```python
from build123d import *

# Parameters (mm, degrees)
SKETCH_1_W          = 55
SKETCH_1_H          = 40
SKETCH_1_R          = 1.5
EXTRUDE_1_DEPTH     = 3
SKETCH_2_W          = 40
SKETCH_2_H          = 3
EXTRUDE_2_DEPTH     = 4
CUT_EXTRUDE_1_REACH = 39.433
SKETCH_3_R          = 1.5
SKETCH_4_R          = 10.5
EXTRUDE_3_DEPTH     = 5
CUT_EXTRUDE_4_REACH = 40.646
CUT_EXTRUDE_START   = -1
SKETCH_5_W          = 41.614213562
SKETCH_5_H          = 21.814213562
SKETCH_6_R          = 1.5
EXTRUDE_5_DEPTH     = 27
SKETCH_7_W          = 6
SKETCH_7_H          = 25
SKETCH_7_R          = 1.5
EXTRUDE_6_DEPTH     = 8
CUT_EXTRUDE_5_REACH = 70.124
SKETCH_8_W          = 8
SKETCH_8_H          = 7.8
FILLET_1_R          = 3
FILLET_2_R          = 3
CUT_EXTRUDE_START_2 = -5
SKETCH_9_R          = 10.5
CUT_EXTRUDE_6_DEPTH = 5
SKETCH_10_W         = 41.614213562
SKETCH_10_H         = 3
EXTRUDE_7_DEPTH     = 18
FILLET_3_R          = 3
CUT_EXTRUDE_7_REACH = 57.154


with BuildPart() as part:
    # 草图1 → 凸台-拉伸1 (new body)
    with BuildSketch(Plane(origin=(0, 0, 0), x_dir=(1, 0, 0), z_dir=(0, 1, 0))):
        Rectangle(SKETCH_1_W, SKETCH_1_H)
        with Locations(Location((22.3, 5, 0), (0, 0, 270))):
            Circle(SKETCH_1_R, mode=Mode.SUBTRACT)
        with Locations(Location((22.3, -5, 0), (0, 0, 90))):
            Circle(SKETCH_1_R, mode=Mode.SUBTRACT)
    extrude(amount=EXTRUDE_1_DEPTH)

    # 草图2 → 凸台-拉伸2 (add)
    with BuildSketch(Plane.ZY.offset(27.5)):
        with Locations((0, 1.5)):
            Rectangle(SKETCH_2_W, SKETCH_2_H)
    extrude(amount=EXTRUDE_2_DEPTH)

    # 草图3 → 切除-拉伸1 (cut, up to next)
    with BuildSketch(Plane.XZ, mode=Mode.PRIVATE) as cut_extrude_1_sk1:
        with Locations(Location((-27.3, 5, 0), (0, 0, 270))):
            Circle(SKETCH_3_R)
    cut_extrude_1_tool1 = extrude(cut_extrude_1_sk1.sketch, amount=-CUT_EXTRUDE_1_REACH, mode=Mode.PRIVATE) & part.part
    # 草图3 → 切除-拉伸1 (cut, up to next)
    with BuildSketch(Plane.XZ, mode=Mode.PRIVATE) as cut_extrude_1_sk2:
        with Locations(Location((-27.3, -5, 0), (0, 0, 270))):
            Circle(SKETCH_3_R)
    cut_extrude_1_tool2 = extrude(cut_extrude_1_sk2.sketch, amount=-CUT_EXTRUDE_1_REACH, mode=Mode.PRIVATE) & part.part
    add(cut_extrude_1_tool1.solids().sort_by_distance((-27.3, 0, 5))[0], mode=Mode.SUBTRACT)
    add(cut_extrude_1_tool2.solids().sort_by_distance((-27.3, 0, -5))[0], mode=Mode.SUBTRACT)

    # 草图4 → 凸台-拉伸3 (add)
    with BuildSketch(Plane.XZ):
        with Locations(Location((-12.5, 0, 0), (0, 0, 90))):
            Circle(SKETCH_4_R)
    extrude(amount=EXTRUDE_3_DEPTH)

    # 草图5 → 切除-拉伸4 (cut, up to next)
    with BuildSketch(Plane.XZ.offset(CUT_EXTRUDE_START), mode=Mode.PRIVATE) as cut_extrude_4_sk1:
        with Locations((-2.5, 0)):
            Rectangle(SKETCH_5_W, SKETCH_5_H)
    cut_extrude_4_tool1 = extrude(cut_extrude_4_sk1.sketch, amount=-CUT_EXTRUDE_4_REACH, mode=Mode.PRIVATE) & part.part
    add(cut_extrude_4_tool1.solids().sort_by_distance((-2.5, 1, 0))[0], mode=Mode.SUBTRACT)

    # 草图6 → 凸台-拉伸5 (add)
    # profile 1 of 2: a face of its own
    with BuildSketch(Plane(origin=(0, 3, 0), x_dir=(1, 0, 0), z_dir=(0, 1, 0))):
        with BuildLine():
            Line((-30.3, -5), (-30.3, 5))
            ThreePointArc((-30.3, 5), (-27.3, 8), (-24.3, 5))
            Line((-24.3, 5), (-24.3, -5))
            ThreePointArc((-24.3, -5), (-27.3, -8), (-30.3, -5))
        make_face()
        with Locations(Location((-27.3, -5, 0), (0, 0, 90))):
            Circle(SKETCH_6_R, mode=Mode.SUBTRACT)
        with Locations(Location((-27.3, 5, 0), (0, 0, 90))):
            Circle(SKETCH_6_R, mode=Mode.SUBTRACT)
    # profile 2 of 2: a face of its own
    with BuildSketch(Plane(origin=(0, 3, 0), x_dir=(1, 0, 0), z_dir=(0, 1, 0))):
        with BuildLine():
            Line((19.3, -5), (19.3, 5))
            ThreePointArc((19.3, 5), (22.3, 8), (25.3, 5))
            Line((25.3, 5), (25.3, -5))
            ThreePointArc((25.3, -5), (22.3, -8), (19.3, -5))
        make_face()
        with Locations(Location((22.3, 5, 0), (0, 0, 270))):
            Circle(SKETCH_6_R, mode=Mode.SUBTRACT)
        with Locations(Location((22.3, -5, 0), (0, 0, 90))):
            Circle(SKETCH_6_R, mode=Mode.SUBTRACT)
    extrude(amount=EXTRUDE_5_DEPTH)

    # 草图7 → 凸台-拉伸6 (add)
    with BuildSketch(Plane(origin=(0, 3, 0), x_dir=(1, 0, 0), z_dir=(0, 1, 0))):
        with Locations((-27.3, 0)):
            Rectangle(SKETCH_7_W, SKETCH_7_H)
        with Locations(Location((-27.3, -5, 0), (0, 0, 90))):
            Circle(SKETCH_7_R, mode=Mode.SUBTRACT)
        with Locations(Location((-27.3, 5, 0), (0, 0, 90))):
            Circle(SKETCH_7_R, mode=Mode.SUBTRACT)
    extrude(amount=EXTRUDE_6_DEPTH)

    # 草图8 → 切除-拉伸5 (cut, up to next)
    with BuildSketch(Plane.ZY.offset(30.3), mode=Mode.PRIVATE) as cut_extrude_5_sk1:
        with Locations((0, 6.9)):
            Rectangle(SKETCH_8_W, SKETCH_8_H)
    cut_extrude_5_tool1 = extrude(cut_extrude_5_sk1.sketch, amount=-CUT_EXTRUDE_5_REACH, mode=Mode.PRIVATE) & part.part
    add(cut_extrude_5_tool1.solids().sort_by_distance((-30.3, 6.9, 0))[0], mode=Mode.SUBTRACT)

    # 圆角1
    fillet_1_edges = [part.edges().sort_by_distance(p)[0] for p in [
        (-27.3, 11, 8),
    ]]
    fillet(fillet_1_edges, radius=FILLET_1_R)

    # 圆角2
    fillet_2_edges = [part.edges().sort_by_distance(p)[0] for p in [
        (-27.3, 11, -8),
    ]]
    fillet(fillet_2_edges, radius=FILLET_2_R)

    # 草图9 → 切除-拉伸6 (cut)
    with BuildSketch(Plane.XZ.offset(5).offset(CUT_EXTRUDE_START_2)):
        with Locations((-12.5, 0)):
            Circle(SKETCH_9_R)
    extrude(amount=CUT_EXTRUDE_6_DEPTH, mode=Mode.SUBTRACT)

    # 草图10 → 凸台-拉伸7 (add)
    with BuildSketch(Plane(origin=(0, 3, 0), x_dir=(1, 0, 0), z_dir=(0, 1, 0))):
        with Locations((-2.5, 12.407106781)):
            Rectangle(SKETCH_10_W, SKETCH_10_H)
        with Locations((-2.5, -12.407106781)):
            Rectangle(SKETCH_10_W, SKETCH_10_H)
    extrude(amount=EXTRUDE_7_DEPTH)

    # 圆角3
    fillet_3_edges = [part.edges().sort_by_distance(p)[0] for p in [
        (-23.307106781, 21, -12.407106781),
        (18.307106781, 21, -12.407106781),
        (18.307106781, 21, 12.407106781),
        (-23.307106781, 21, 12.407106781),
    ]]
    fillet(fillet_3_edges, radius=FILLET_3_R)

    # 切除-拉伸7: up to this face of the body (flat: up to its plane)
    cut_extrude_7_end = Plane(part.part.faces().sort_by_distance((-2.5, 11.956820585, -13.907106781))[0])
    # 草图11 → 切除-拉伸7 (cut, up to the picked face)
    with BuildSketch(Plane.XY.offset(13.907106781), mode=Mode.PRIVATE) as cut_extrude_7_sk1:
        with BuildLine():
            Line((-15.307106781, 14.245523658), (10.307106781, 14.245523658))
            ThreePointArc((10.307106781, 14.245523658), (14.052630439, 10.5), (10.307106781, 6.754476342))
            Line((10.307106781, 6.754476342), (-15.307106781, 6.754476342))
            ThreePointArc((-15.307106781, 6.754476342), (-19.052630439, 10.5), (-15.307106781, 14.245523658))
        make_face()
    cut_extrude_7_tool1 = split(extrude(cut_extrude_7_sk1.sketch, amount=-CUT_EXTRUDE_7_REACH, mode=Mode.PRIVATE), bisect_by=cut_extrude_7_end, keep=Keep.BOTH, mode=Mode.PRIVATE)
    add(cut_extrude_7_tool1.solids().sort_by(Axis((-2.5, 10.5, 13.907107), (0, 0, -1)))[0], mode=Mode.SUBTRACT)


solid = part.part
```
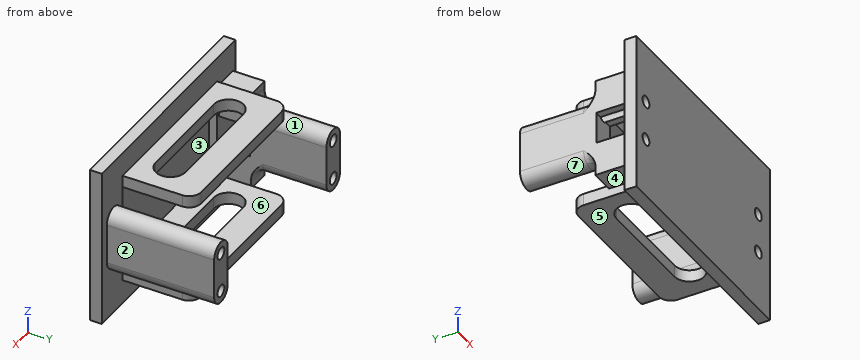
Can you work these out from the model? Positions are in its coordinate system, mm. Face numbers are marked on the shaded views. A direction names the side the tool comes from. Give positions to 0.01 mm unless a question says otherwise; leave off trailing zeros. Order: outer loops, then holes, each group sorted by start corner. A loop starts at its lowest first (then second) coordinate and runs counter-clockwise, first axis right, second up. Notation, with made-up numbers: (39.5, -37) - (84.5, -37) arc R16 ccw to (84.5, -8) - close; hole circle Ø11 at (-4.5, 6). An arc over 180 degrees is marked (long way). Use a Markdown table: item, result. Add a question column.
Q1. I'm going to push flat-ended pins straight in: pin 1 (2.5 mm diameter, centred on y = 10, z = 12.5, fed in from +X); pin 2 (0.9 mm diameter, centred on x = -25.5, y = 6.5, fed in from +Z); pin 3 (1 mm diameter, centred on x = 8.5, y = 4, fed in from +Z); pin 4 (1.5 mm diameter, centred on x = 7, y = 11.5, fed in from -Z). Where does each tip first touch, or does it pass through?
Q2. If we section it at D-D on y = 22: Write out the boundary of the cut face in (x, z).
Q3. If we section it at A-A on y = 16: Write out the boundary of the cut face in (x, z).
Q4. If we mould it in two halves opening along Z, with no side actions, what happens to the marked faces 1, 2 and 3? For each: released by +Z, released by -Z, zero draft, split by the parting line, or undercut.
Q5. If we section it at B-B on x = 22.3: Write out the boundary of the cut face in (y, z), plus the area to 3 significant figures.
Q6. Please list where these lines run through material, in increasing order: line 1 along X through (y, z) = (21.5, -5); line 2 along Z through (x, y) = (22, 15); line 3 along Z through (x, y) = (1, 19.5).
Q7. If we section it at C-C on z = -1.5: Write out the boundary of the cut face in (x, y), plus the area to 3 significant figures.
Q8. On a 3-axis mill with a long thin cutter (end or side, diameter ignored), from which of +Z, -Z, +X, -X, +Y, -Y can I reach the whole of each face in a straight line? I mean the marked faces 4, 5, 6 and 7. Say none if no direction works.
Answers follow:
| question | item | result |
|---|---|---|
| 1 | pin 1 | stops at x = 18.31 |
| 1 | pin 2 | stops at z = 12.5 |
| 1 | pin 3 | stops at z = 13.91 |
| 1 | pin 4 | passes through |
| 2 | outline | (-30.3, -5) arc R3 ccw to (-24.3, -5) - (-24.3, 5) arc R3 ccw to (-30.3, 5) - close; (19.3, -5) arc R3 ccw to (25.3, -5) - (25.3, 5) arc R3 ccw to (19.3, 5) - close; hole circle Ø3 at (-27.3, -5); hole circle Ø3 at (-27.3, 5); hole circle Ø3 at (22.3, -5); hole circle Ø3 at (22.3, 5) |
| 3 | outline | (-30.3, -5) arc R3 ccw to (-24.3, -5) - (-24.3, 5) arc R3 ccw to (-30.3, 5) - close; (-23.31, -13.91) - (18.31, -13.91) - (18.31, -10.91) - (-23.31, -10.91) - close; (-23.31, 10.91) - (18.31, 10.91) - (18.31, 13.91) - (-23.31, 13.91) - close; (19.3, -5) arc R3 ccw to (25.3, -5) - (25.3, 5) arc R3 ccw to (19.3, 5) - close; hole circle Ø3 at (-27.3, -5); hole circle Ø3 at (-27.3, 5); hole circle Ø3 at (22.3, -5); hole circle Ø3 at (22.3, 5) |
| 4 | face 1 | released by +Z |
| 4 | face 2 | zero draft |
| 4 | face 3 | undercut |
| 5 | outline | (0, -20) - (3, -20) - (3, -8) - (30, -8) - (30, -6.5) - (0, -6.5) - close; (0, -3.5) - (30, -3.5) - (30, 3.5) - (0, 3.5) - close; (0, 6.5) - (30, 6.5) - (30, 8) - (3, 8) - (3, 20) - (0, 20) - close |
| 5 | area | 372 mm^2 |
| 6 | line 1 | x = -30.3 to -28.8, -25.8 to -24.3, 19.3 to 20.8, 23.8 to 25.3 |
| 6 | line 2 | z = -7.98 to -6.47, -3.53 to 3.53, 6.47 to 7.98 |
| 6 | line 3 | z = -13.91 to -10.91, 10.91 to 13.91 |
| 7 | outline | (-31.5, 0) - (27.5, 0) - (27.5, 3) - (25.3, 3) - (25.3, 30) - (19.3, 30) - (19.3, 3) - (18.31, 3) - (18.31, 1) - (-23.31, 1) - (-23.31, 3) - (-31.5, 3) - close; (-30.3, 10.8) - (-24.3, 10.8) - (-24.3, 30) - (-30.3, 30) - close |
| 7 | area | 371 mm^2 |
| 8 | face 4 | -Z, -X, +Y |
| 8 | face 5 | -Z, +X, -X, +Y |
| 8 | face 6 | +Y |
| 8 | face 7 | -Z, +Y |
